Build history of the part. All positions in model axes, mm. Coordinates: 2 decimals unless noted, no trailing zeros. Write each question's results on one line, items separated by ' | '.
from build123d import *

# Parameters (mm, degrees)
SKETCH1_W           = 714.375
SKETCH1_H           = 274.6375
BOSS_EXTRUDE1_DEPTH = 4.7625
CUT_EXTRUDE1_DEPTH  = 5.7625
CUT_EXTRUDE3_DEPTH  = 5.7625
CUT_EXTRUDE4_REACH  = 6.763
SKETCH5_R           = 2.15265


with BuildPart() as part:
    # Sketch1 → Boss-Extrude1 (new body)
    with BuildSketch(Plane.XY):
        Rectangle(SKETCH1_W, SKETCH1_H)
    extrude(amount=BOSS_EXTRUDE1_DEPTH)

    # Sketch2 → Cut-Extrude1 (cut, through all)
    with BuildSketch(Plane.XY.offset(4.7625)):
        with BuildLine():
            Line((12.285980323, -89.570459076), (10.351389114, -91.505050285))
            ThreePointArc((10.351389114, -91.505050285), (0, -88.10625), (-10.351389114, -91.505050285))
            Line((-10.351389114, -91.505050285), (-12.285980323, -89.570459076))
            ThreePointArc((-12.285980323, -89.570459076), (-15.998290924, -89.570459076), (-15.998290924, -93.282769677))
            Line((-15.998290924, -93.282769677), (-14.063699715, -95.217360886))
            ThreePointArc((-14.063699715, -95.217360886), (-17.4625, -105.56875), (-14.063699715, -115.920139114))
            Line((-14.063699715, -115.920139114), (-15.998290924, -117.854730323))
            ThreePointArc((-15.998290924, -117.854730323), (-15.998290924, -121.567040924), (-12.285980323, -121.567040924))
            Line((-12.285980323, -121.567040924), (-10.351389114, -119.632449715))
            ThreePointArc((-10.351389114, -119.632449715), (0, -123.03125), (10.351389114, -119.632449715))
            Line((10.351389114, -119.632449715), (12.285980323, -121.567040924))
            ThreePointArc((12.285980323, -121.567040924), (15.998290924, -121.567040924), (15.998290924, -117.854730323))
            Line((15.998290924, -117.854730323), (14.063699715, -115.920139114))
            ThreePointArc((14.063699715, -115.920139114), (17.4625, -105.56875), (14.063699715, -95.217360886))
            Line((14.063699715, -95.217360886), (15.998290924, -93.282769677))
            ThreePointArc((15.998290924, -93.282769677), (15.998290924, -89.570459076), (12.285980323, -89.570459076))
        make_face()
        with BuildLine():
            Line((-305.214019677, -89.570459076), (-307.148610886, -91.505050285))
            ThreePointArc((-307.148610886, -91.505050285), (-317.5, -88.10625), (-327.851389114, -91.505050285))
            Line((-327.851389114, -91.505050285), (-329.785980323, -89.570459076))
            ThreePointArc((-329.785980323, -89.570459076), (-333.498290924, -89.570459076), (-333.498290924, -93.282769677))
            Line((-333.498290924, -93.282769677), (-331.563699715, -95.217360886))
            ThreePointArc((-331.563699715, -95.217360886), (-334.9625, -105.56875), (-331.563699715, -115.920139114))
            Line((-331.563699715, -115.920139114), (-333.498290924, -117.854730323))
            ThreePointArc((-333.498290924, -117.854730323), (-333.498290924, -121.567040924), (-329.785980323, -121.567040924))
            Line((-329.785980323, -121.567040924), (-327.851389114, -119.632449715))
            ThreePointArc((-327.851389114, -119.632449715), (-317.5, -123.03125), (-307.148610886, -119.632449715))
            Line((-307.148610886, -119.632449715), (-305.214019677, -121.567040924))
            ThreePointArc((-305.214019677, -121.567040924), (-301.501709076, -121.567040924), (-301.501709076, -117.854730323))
            Line((-301.501709076, -117.854730323), (-303.436300285, -115.920139114))
            ThreePointArc((-303.436300285, -115.920139114), (-300.0375, -105.56875), (-303.436300285, -95.217360886))
            Line((-303.436300285, -95.217360886), (-301.501709076, -93.282769677))
            ThreePointArc((-301.501709076, -93.282769677), (-301.501709076, -89.570459076), (-305.214019677, -89.570459076))
        make_face()
        with BuildLine():
            Line((329.785980323, -89.570459076), (327.851389114, -91.505050285))
            ThreePointArc((327.851389114, -91.505050285), (317.5, -88.10625), (307.148610886, -91.505050285))
            Line((307.148610886, -91.505050285), (305.214019677, -89.570459076))
            ThreePointArc((305.214019677, -89.570459076), (301.501709076, -89.570459076), (301.501709076, -93.282769677))
            Line((301.501709076, -93.282769677), (303.436300285, -95.217360886))
            ThreePointArc((303.436300285, -95.217360886), (300.0375, -105.56875), (303.436300285, -115.920139114))
            Line((303.436300285, -115.920139114), (301.501709076, -117.854730323))
            ThreePointArc((301.501709076, -117.854730323), (301.501709076, -121.567040924), (305.214019677, -121.567040924))
            Line((305.214019677, -121.567040924), (307.148610886, -119.632449715))
            ThreePointArc((307.148610886, -119.632449715), (317.5, -123.03125), (327.851389114, -119.632449715))
            Line((327.851389114, -119.632449715), (329.785980323, -121.567040924))
            ThreePointArc((329.785980323, -121.567040924), (333.498290924, -121.567040924), (333.498290924, -117.854730323))
            Line((333.498290924, -117.854730323), (331.563699715, -115.920139114))
            ThreePointArc((331.563699715, -115.920139114), (334.9625, -105.56875), (331.563699715, -95.217360886))
            Line((331.563699715, -95.217360886), (333.498290924, -93.282769677))
            ThreePointArc((333.498290924, -93.282769677), (333.498290924, -89.570459076), (329.785980323, -89.570459076))
        make_face()
    extrude(amount=-CUT_EXTRUDE1_DEPTH, mode=Mode.SUBTRACT)

    # Sketch4 → Cut-Extrude3 (cut, through all)
    with BuildSketch(Plane.XY.offset(4.7625)):
        with BuildLine():
            Line((277.1521, 88.42375), (277.1521, 97.31375))
            ThreePointArc((277.1521, 97.31375), (279.4, 99.56165), (281.6479, 97.31375))
            Line((281.6479, 97.31375), (281.6479, 88.42375))
            ThreePointArc((281.6479, 88.42375), (279.4, 86.17585), (277.1521, 88.42375))
        make_face()
        with BuildLine():
            Line((-277.1521, 88.42375), (-277.1521, 97.31375))
            ThreePointArc((-277.1521, 97.31375), (-279.4, 99.56165), (-281.6479, 97.31375))
            Line((-281.6479, 97.31375), (-281.6479, 88.42375))
            ThreePointArc((-281.6479, 88.42375), (-279.4, 86.17585), (-277.1521, 88.42375))
        make_face()
    extrude(amount=-CUT_EXTRUDE3_DEPTH, mode=Mode.SUBTRACT)

    # Sketch5 → Cut-Extrude4 (cut, up to next)
    with BuildSketch(Plane.XY.offset(4.7625), mode=Mode.PRIVATE) as cut_extrude4_sk1:
        with Locations((-127, -105.56875)):
            Circle(SKETCH5_R)
    cut_extrude4_tool1 = extrude(cut_extrude4_sk1.sketch, amount=-CUT_EXTRUDE4_REACH, mode=Mode.PRIVATE) & part.part
    add(cut_extrude4_tool1.solids().sort_by_distance((-127, -105.56875, 4.7625))[0], mode=Mode.SUBTRACT)
    # Sketch5 → Cut-Extrude4 (cut, up to next)
    with BuildSketch(Plane.XY.offset(4.7625), mode=Mode.PRIVATE) as cut_extrude4_sk2:
        with Locations((-215.9, -105.56875)):
            Circle(SKETCH5_R)
    cut_extrude4_tool2 = extrude(cut_extrude4_sk2.sketch, amount=-CUT_EXTRUDE4_REACH, mode=Mode.PRIVATE) & part.part
    add(cut_extrude4_tool2.solids().sort_by_distance((-215.9, -105.56875, 4.7625))[0], mode=Mode.SUBTRACT)
    # Sketch5 → Cut-Extrude4 (cut, up to next)
    with BuildSketch(Plane.XY.offset(4.7625), mode=Mode.PRIVATE) as cut_extrude4_sk3:
        with Locations((215.9, -105.56875)):
            Circle(SKETCH5_R)
    cut_extrude4_tool3 = extrude(cut_extrude4_sk3.sketch, amount=-CUT_EXTRUDE4_REACH, mode=Mode.PRIVATE) & part.part
    add(cut_extrude4_tool3.solids().sort_by_distance((215.9, -105.56875, 4.7625))[0], mode=Mode.SUBTRACT)
    # Sketch5 → Cut-Extrude4 (cut, up to next)
    with BuildSketch(Plane.XY.offset(4.7625), mode=Mode.PRIVATE) as cut_extrude4_sk4:
        with Locations((127, -105.56875)):
            Circle(SKETCH5_R)
    cut_extrude4_tool4 = extrude(cut_extrude4_sk4.sketch, amount=-CUT_EXTRUDE4_REACH, mode=Mode.PRIVATE) & part.part
    add(cut_extrude4_tool4.solids().sort_by_distance((127, -105.56875, 4.7625))[0], mode=Mode.SUBTRACT)


solid = part.part
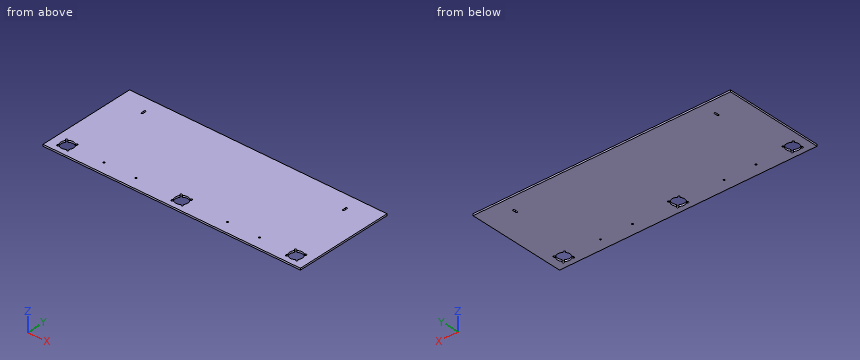
1. Band-saw the part on A-A on z = 1.6. Give the number of separate pieces and of enclosed holes in the cut face, then the cut area to 3 significant figures.
Solved:
separate pieces: 1 | enclosed holes: 9 | area: 193,000 mm2
2. Drop a flat-ended pin along its axis: pin 1 Ø5.5 at (x, y) = (-215.9, -105.57) entering from +Z. Give the stop position or say it passes through.
Solved:
pin 1: stops at z = 4.76
3. Probe line 1 (X direction, y = 96.5, z = 2.5); line 2 (Y direction, x = 127, z = 2.8); line 3 (X direction, y = -108.5, z = 4.4). List the from-to ranges inside material, lowest first.
Solved:
line 1: x = -357.19 to -281.65, -277.15 to 277.15, 281.65 to 357.19 | line 2: y = -137.32 to -107.72, -103.42 to 137.32 | line 3: x = -357.19 to -334.71, -300.29 to -17.21, 17.21 to 300.29, 334.71 to 357.19
